from build123d import *

# Parameters (mm, degrees)
F0_R      = 11.5
F1_DEPTH  = 2
F3_DEPTH  = 77
F5_DEPTH  = 3
F7_DEPTH  = 3
F9_DEPTH  = 5
F11_DEPTH = 3
F12_R     = 19
F13_DEPTH = 8
F14_R     = 19
F15_DEPTH = 40
F16_W     = 52
F16_H     = 3
F17_DEPTH = 38.5
F19_DEPTH = 3
F21_DEPTH = 10
F22_W     = 3
F22_H     = 38.5
F23_DEPTH = 5
F25_R     = 2.5
F25_W     = 47
F25_H     = 2
F26_DEPTH = 5
F27_DEPTH = 1
F29_DEPTH = 75
F30_DEPTH = 2


with BuildPart() as f1:
    # F0 (on Front) → F1 (new body)
    with BuildSketch(Plane.XZ):
        with BuildLine():
            Line((26, 36), (-26, 36))
            ThreePointArc((-26, 36), (-33.0710678119, 33.0710678119), (-36, 26))
            Line((-36, 26), (-36, -26))
            ThreePointArc((-36, -26), (-33.0710678119, -33.0710678119), (-26, -36))
            Line((-26, -36), (26, -36))
            ThreePointArc((26, -36), (33.0710678119, -33.0710678119), (36, -26))
            Line((36, -26), (36, 26))
            ThreePointArc((36, 26), (33.0710678119, 33.0710678119), (26, 36))
        make_face()
        with BuildLine():
            Line((24, -34), (-24, -34))
            ThreePointArc((-24, -34), (-31.0710678119, -31.0710678119), (-34, -24))
            Line((-34, -24), (-34, 24))
            ThreePointArc((-34, 24), (-31.0710678119, 31.0710678119), (-24, 34))
            Line((-24, 34), (24, 34))
            ThreePointArc((24, 34), (31.0710678119, 31.0710678119), (34, 24))
            Line((34, 24), (34, -24))
            ThreePointArc((34, -24), (31.0710678119, -31.0710678119), (24, -34))
        make_face(mode=Mode.SUBTRACT)
        with BuildLine():
            ThreePointArc((-34, -24), (-31.0710678119, -31.0710678119), (-24, -34))
            Line((-24, -34), (24, -34))
            ThreePointArc((24, -34), (31.0710678119, -31.0710678119), (34, -24))
            Line((34, -24), (34, 24))
            ThreePointArc((34, 24), (31.0710678119, 31.0710678119), (24, 34))
            Line((24, 34), (-24, 34))
            ThreePointArc((-24, 34), (-31.0710678119, 31.0710678119), (-34, 24))
            Line((-34, 24), (-34, -24))
        make_face()
        Circle(F0_R, mode=Mode.SUBTRACT)
    extrude(amount=F1_DEPTH)

    # F2 (on face) → F3 (join)
    with BuildSketch(Plane.XZ.offset(2)):
        with BuildLine():
            Line((26, 36), (-26, 36))
            ThreePointArc((-26, 36), (-33.0710678119, 33.0710678119), (-36, 26))
            Line((-36, 26), (-36, -26))
            ThreePointArc((-36, -26), (-33.0710678119, -33.0710678119), (-26, -36))
            Line((-26, -36), (26, -36))
            ThreePointArc((26, -36), (33.0710678119, -33.0710678119), (36, -26))
            Line((36, -26), (36, 26))
            ThreePointArc((36, 26), (33.0710678119, 33.0710678119), (26, 36))
        make_face()
        with BuildLine():
            Line((24, -34), (-24, -34))
            ThreePointArc((-24, -34), (-31.0710678119, -31.0710678119), (-34, -24))
            Line((-34, -24), (-34, 24))
            ThreePointArc((-34, 24), (-31.0710678119, 31.0710678119), (-24, 34))
            Line((-24, 34), (24, 34))
            ThreePointArc((24, 34), (31.0710678119, 31.0710678119), (34, 24))
            Line((34, 24), (34, -24))
            ThreePointArc((34, -24), (31.0710678119, -31.0710678119), (24, -34))
        make_face(mode=Mode.SUBTRACT)
    extrude(amount=F3_DEPTH)

    # F4 (on face) → F5 (cut)
    with BuildSketch(Plane(origin=(-36, 0, 0), x_dir=(0, -1, 0), z_dir=(-1, 0, 0))):
        with BuildLine():
            ThreePointArc((62, 13), (58.4852813742, 21.4852813742), (50, 25))
            Line((50, 25), (47, 25))
            ThreePointArc((47, 25), (38.5147186258, 21.4852813742), (35, 13))
            Line((35, 13), (35, -13))
            ThreePointArc((35, -13), (38.5147186258, -21.4852813742), (47, -25))
            Line((47, -25), (50, -25))
            ThreePointArc((50, -25), (58.4852813742, -21.4852813742), (62, -13))
            Line((62, -13), (62, 13))
        make_face()
    extrude(amount=-F5_DEPTH, mode=Mode.SUBTRACT)

    # F6 (on face) → F7 (cut)
    with BuildSketch(Plane.XY.offset(36)):
        with BuildLine():
            Line((19, -30), (19, -22))
            ThreePointArc((19, -22), (0, -3), (-19, -22))
            Line((-19, -22), (-19, -30))
            ThreePointArc((-19, -30), (0, -49), (19, -30))
        make_face()
    extrude(amount=-F7_DEPTH, mode=Mode.SUBTRACT)

    # F8 (on face) → F9 (join)
    with BuildSketch(Plane.XY.offset(36)):
        with BuildLine():
            Line((-20.5, -22), (-20.5, -30))
            ThreePointArc((-20.5, -30), (0, -50.5), (20.5, -30))
            Line((20.5, -30), (20.5, -22))
            ThreePointArc((20.5, -22), (0, -1.5), (-20.5, -22))
        make_face()
        with BuildLine():
            ThreePointArc((-19, -22), (0, -3), (19, -22))
            Line((19, -22), (19, -22.3025978408))
            Line((19, -22.3025978408), (19, -29.6974021592))
            Line((19, -29.6974021592), (19, -30))
            ThreePointArc((19, -30), (0, -49), (-19, -30))
            Line((-19, -30), (-19, -22))
        make_face(mode=Mode.SUBTRACT)
        with BuildLine():
            Line((19, -22.3025978408), (19, -22))
            ThreePointArc((19, -22), (0, -3), (-19, -22))
            Line((-19, -22), (-19, -30))
            ThreePointArc((-19, -30), (0, -49), (19, -30))
            Line((19, -30), (19, -29.6974021592))
            Line((19, -29.6974021592), (19, -22.3025978408))
        make_face()
    extrude(amount=F9_DEPTH)

    # F10 (on face) → F11 (join)
    with BuildSketch(Plane.XY.offset(36)):
        with BuildLine():
            Line((20.5, -30), (20.5, -22))
            ThreePointArc((20.5, -22), (0, -1.5), (-20.5, -22))
            Line((-20.5, -22), (-20.5, -30))
            ThreePointArc((-20.5, -30), (0, -50.5), (20.5, -30))
        make_face()
    extrude(amount=F11_DEPTH)

    # F12 (on face) → F13 (cut)
    with BuildSketch(Plane.XY.offset(41)):
        with Locations((0, -22)):
            Circle(F12_R)
    extrude(amount=-F13_DEPTH, mode=Mode.SUBTRACT)

    # F14 (on face) → F15 (join)
    with BuildSketch(Plane.XY.offset(41)):
        with BuildLine():
            Line((-20.5, -22), (-20.5, -28.4807406984))
            ThreePointArc((-20.5, -28.4807406984), (0, -43.5), (20.5, -28.4807406984))
            Line((20.5, -28.4807406984), (20.5, -22))
            ThreePointArc((20.5, -22), (0, -1.5), (-20.5, -22))
        make_face()
        with Locations((0, -22)):
            Circle(F14_R, mode=Mode.SUBTRACT)
    extrude(amount=F15_DEPTH)

    # F16 (on face) → F17 (join)
    with BuildSketch(Plane(origin=(0, 0, -36), x_dir=(1, 0, 0), z_dir=(0, 0, -1))):
        with Locations((0, 77.5)):
            Rectangle(F16_W, F16_H)
    extrude(amount=F17_DEPTH)

    # F18 (on face) → F19 (cut)
    with BuildSketch(Plane(origin=(0, 0, -36), x_dir=(1, 0, 0), z_dir=(0, 0, -1))):
        with BuildLine():
            Line((-17, 12), (17, 12))
            ThreePointArc((17, 12), (23.3298247558, 33), (17, 54))
            Line((17, 54), (-17, 54))
            ThreePointArc((-17, 54), (-23.3298247558, 33), (-17, 12))
        make_face()
    extrude(amount=-F19_DEPTH, mode=Mode.SUBTRACT)

    # F20 (on face) → F21 (join)
    with BuildSketch(Plane(origin=(0, 0, -36), x_dir=(1, 0, 0), z_dir=(0, 0, -1))):
        with BuildLine():
            ThreePointArc((19, 50.6158820109), (23.3298247558, 33), (19, 15.3841179891))
            Line((19, 15.3841179891), (19, 10))
            ThreePointArc((19, 10), (23.2866263695, 16.8090036252), (26, 24.3836521016))
            Line((26, 24.3836521016), (26, 41.6163478984))
            ThreePointArc((26, 41.6163478984), (23.2866263695, 49.1909963748), (19, 56))
            Line((19, 56), (19, 50.6158820109))
        make_face()
        with BuildLine():
            Line((-19, 56), (-19, 50.6158820109))
            ThreePointArc((-19, 50.6158820109), (-18.0437883513, 52.3338197434), (-17, 54))
            Line((-17, 54), (17, 54))
            ThreePointArc((17, 54), (18.0437883513, 52.3338197434), (19, 50.6158820109))
            Line((19, 50.6158820109), (19, 56))
            Line((19, 56), (-19, 56))
        make_face()
        with BuildLine():
            Line((-19, 10), (-19, 15.3841179891))
            ThreePointArc((-19, 15.3841179891), (-23.3298247558, 33), (-19, 50.6158820109))
            Line((-19, 50.6158820109), (-19, 56))
            ThreePointArc((-19, 56), (-23.2866263695, 49.1909963748), (-26, 41.6163478984))
            Line((-26, 41.6163478984), (-26, 24.3836521016))
            ThreePointArc((-26, 24.3836521016), (-23.2866263695, 16.8090036252), (-19, 10))
        make_face()
        with BuildLine():
            Line((17, 12), (-17, 12))
            ThreePointArc((-17, 12), (-18.0437883513, 13.6661802566), (-19, 15.3841179891))
            Line((-19, 15.3841179891), (-19, 10))
            Line((-19, 10), (19, 10))
            Line((19, 10), (19, 15.3841179891))
            ThreePointArc((19, 15.3841179891), (18.0437883513, 13.6661802566), (17, 12))
        make_face()
    extrude(amount=F21_DEPTH)

    # F22 (on face) → F23 (join)
    with BuildSketch(Plane.YZ.offset(26)):
        Polygon((-76, -36), (-76, -74.5), (-69, -74.5), (-59, -36), align=None)
        with Locations((-77.5, -55.25)):
            Rectangle(F22_W, F22_H)
    extrude(amount=-F23_DEPTH)

    # F25 (on face) → F26 (join)
    with BuildSketch(Plane(origin=(0, 0, -74.5), x_dir=(1, 0, 0), z_dir=(0, 0, -1))):
        with BuildLine():
            Line((37, 74), (26, 74))
            Line((26, 74), (21, 74))
            Line((21, 74), (-26, 74))
            Line((-26, 74), (-37, 74))
            ThreePointArc((-37, 74), (-42, 69), (-37, 64))
            Line((-37, 64), (37, 64))
            ThreePointArc((37, 64), (42, 69), (37, 74))
        make_face()
        with Locations((-37, 69)):
            Circle(F25_R, mode=Mode.SUBTRACT)
        with Locations((0, 69)):
            Circle(F25_R, mode=Mode.SUBTRACT)
        with Locations((37, 69)):
            Circle(F25_R, mode=Mode.SUBTRACT)
        Polygon((26, 79), (-26, 79), (-26, 76), (21, 76), (21, 74), (26, 74), align=None)
        with Locations((-2.5, 75)):
            Rectangle(F25_W, F25_H)
        with BuildLine():
            Line((-26.0336585343, 79), (-26, 79))
            Line((-26, 79), (26, 79))
            Line((26, 79), (26, 84))
            ThreePointArc((26, 84), (24.5355339059, 87.5355339059), (21, 89))
            Line((21, 89), (-21.0336585343, 89))
            ThreePointArc((-21.0336585343, 89), (-24.5691924402, 87.5355339059), (-26.0336585343, 84))
            Line((-26.0336585343, 84), (-26.0336585343, 79))
        make_face()
        with Locations((0, 84)):
            Circle(F25_R, mode=Mode.SUBTRACT)
    extrude(amount=-F26_DEPTH)

    # F27 (add): faces of the model
    f27_faces = [f1.faces().sort_by_distance(p)[0] for p in [
        (23.5, -77.5, -74.5),
        (-2.5, -77.5, -74.5),
        (23.5, -72.5, -74.5),
        (-26.0168292671, -79.5298586246, -74.5),
        (-41.1514718626, -69, -74.5),
    ]]
    extrude(f27_faces, amount=F27_DEPTH)

    # F28 (on face) → F29 (cut)
    with BuildSketch(Plane.YZ.offset(36)):
        with BuildLine():
            Line((-78, 5), (-79, 5))
            Line((-79, 5), (-79, -22))
            Line((-79, -22), (-78, -22))
            ThreePointArc((-78, -22), (-74.4644660941, -20.5355339059), (-73, -17))
            Line((-73, -17), (-73, 0))
            ThreePointArc((-73, 0), (-74.4644660941, 3.5355339059), (-78, 5))
        make_face()
    extrude(amount=-F29_DEPTH, mode=Mode.SUBTRACT)

    # F30 (add): a face of the model
    f30_faces = [f1.faces().sort_by_distance(p)[0] for p in [
        (-0.0056811519, -75.1326620312, -75.5),
    ]]
    extrude(f30_faces, amount=F30_DEPTH)


solid = f1.part
Source: CAD feature listing. Evaluate the final solid. Frame: model axes, mm. A direction names the side the tool comes from. Give positions to 0.01 mm unless a question says otherwise; leave off trailing zeros. Write each loop counter-clockwise with the first axis right and the second up, starting at its lowest first coordinate (ties: lowest second). Pieces come first, ordered by that corner, then holes. Notation, with made-up numbers: (-24, 44.5) - (25, 44.5) arc R17 ccw to (25, 66.5) - close; hole circle Ø10 at (-14.75, 86). An arc over 180 degrees is marked (long way). Write item = value, one per line. Start each with the question number.
Q1. Cut plane B-B, the plane x = -28. Return loops of the section in (y, z), then the cut area to 3 significant figures.
Q2. Draft query along Y for faces 4 (the cylindrical face through (-34.99, -38.61, 21.58)), 5 (the flat face through (0, -11, -46)), 6 (the cylindrical face through (23.24, -16.71, -40.93)). Return one class per face: +Y half, -Y half, draft (parallel to the pull), parting line (faces both ways), or undercut.
Q3. Reachability of faces 1 (the flat face through (-0.2, -79, 34.4)), 2 (the cylindrical face through (-35, -74, 3)), 3 (the flat face through (15, -2, 0)) from +Z, -Z, +X, -X, +Y, -Y: full face, straight path, thin tool, end or side. Return the list, or none.
Q4. Cut plane C-C, the plane z = 49.5. Return loops of the section in (x, y).
Q5. Pin query (flat end, axial travel): pin 1 Ø6 at (x, y) = (-37, -69) entering from +Z; pin 2 Ø6 at (y, z) = (-65, -26) entering from -X; pin 3 Ø2 at (y, z) = (-32.5, 58) entering from +X; pin 4 Ø6 at (x, y) = (-12, -29.5) entering from +Z. Return the tip coordinate at first contact, or that it passes through.
Q6. Cut plane A-A, the plane z = -8.5. Return loops of the section in (x, y).
Q7. Cut plane D-D, the plane x = 0. Give the number of separate pieces and of enclosed holes in the cut face, then the cut area to 4 significant figures.
Q8. Material intervals for probe 1 along Y at (x, z) = (0, -73.75); probe 2 along X at (y, z) = (-69, -71.25); probe 3 along Z at (x, y) = (17.5, -67.5), sorted ascending.
Computed values:
q1.outline = (-79, -35.8) - (0, -35.8) - (0, 35.8) - (-79, 35.8) - (-79, 33.17) - (-2, 33.17) - (-2, -33.17) - (-79, -33.17) - close; (-74, -77.5) - (-64, -77.5) - (-64, -69.5) - (-74, -69.5) - close
q1.area = 629 mm²
q2.face_4 = undercut
q2.face_5 = draft
q2.face_6 = +Y half
q3.face_1 = +Z, +X, -X, -Y
q3.face_2 = +X, -X, -Y
q3.face_3 = -Y
q4.outline = (-20.5, -28.48) arc R21.5 ccw to (20.5, -28.48) - (20.5, -22) arc R20.5 ccw to (-20.5, -22) - close; hole circle Ø38 at (0, -22)
q5.pin_1 = 32
q5.pin_2 = -36
q5.pin_3 = 19.29
q5.pin_4 = through
q6.outline = (-36, -73) - (-34, -73) - (-34, -62) - (-36, -62) - close; (-36, -35) - (-34, -35) - (-34, -2) - (-7.75, -2) - (-7.75, 0) - (-36, 0) - close; (7.75, -2) - (34, -2) - (34, -73) - (36, -73) - (36, 0) - (7.75, 0) - close
q7.separate_pieces = 6
q7.enclosed_holes = 0
q7.area = 705.5 mm²
q8.probe_1 = -89 to -86.5, -81.5 to -71.5, -66.5 to -64
q8.probe_2 = -42 to -39.5, -34.5 to -2.5, 2.5 to 34.5, 39.5 to 42
q8.probe_3 = -77.5 to -69.5, -36 to -34, 34 to 36
